Design review of the part built by this model. Coordinates are the model's own, in mm. A direction names the side the tool comes from. Coordinates: 2 decimals unless noted, no trailing zeros. Order: outer loops, then holes, each group sorted by start corner. A loop starts at its lowest first (then second) coordinate and runs counter-clockwise, first axis right, second up.
from build123d import *

# Parameters (mm, degrees)
BASE_EXTRUDE_THIN_DEPTH = 30
CHAMFER1_SIZE           = 1.4
CHAMFER1_SIZE2          = 0.808290377


with BuildPart() as part:
    # Sketch1 → Base-Extrude-Thin (new, symmetric)
    with BuildSketch(Plane.XY):
        with BuildLine():
            ThreePointArc((-0.5, 2.958039892), (0, -3), (0.5, 2.958039892))
            Line((0.5, 2.958039892), (0.3, 1.774823935))
            ThreePointArc((0.3, 1.774823935), (0, -1.8), (-0.3, 1.774823935))
            Line((-0.3, 1.774823935), (-0.5, 2.958039892))
        make_face()
    extrude(amount=BASE_EXTRUDE_THIN_DEPTH, both=True)

    # Chamfer1
    chamfer1_edges = [part.edges().sort_by_distance(p)[0] for p in [
        (0, -3, 30),
        (0, -3, -30),
    ]]
    chamfer1_side = [part.faces().sort_by_distance(p)[0] for p in [
        (0, -3, 0),
    ]]
    chamfer(chamfer1_edges, length=CHAMFER1_SIZE, length2=CHAMFER1_SIZE2, reference=chamfer1_side[0])


solid = part.part
1. Add section B-B (z = -19.5). Give the boundary of the cut face in (x, y).
2. Add section A-A (y = 0). Give the boundary of the cut face in (x, z).
3. Insertion check: pin 1 (1 mm diameter, centred on x = 1.5, z = -9.5, fed in from +Y); pin 2 (1.5 mm diameter, centred on y = -1.5, z = -14, fed in from +X). Each pin has a flat end and moves straight along its axis. Give the tip position at first contact, or say it passes through.
4. For faces 5 (the flat face through (0, -2, 30)), 6 (the flat face through (-0.4, 2.36, 0.42)), list the 3-axis set-ups (+Z, -Z, +X, -X, +Y, -Y) from which the entire face can be reached by the end or side of a thin tool; tool diameter is ignored.
5. Mouldability with a two-part tool opening along X and no side actions: class faces 1 (the cylindrical face through (0.07, -1.8, 0.42)), 2 (the flat face through (0, -2, -30)), 3 (the conical face through (-0.097, -2.319, 29.776)), 4 (the flat face through (0.4, 2.37, 0.42)) as pulls with the +X half, pulls with the -X half, needs draft (parallel to the pull), parting line crosses it, or undercut.
6. To check wall thickness, follow line 1 (X direction, y = 0, z = -5); line 2 (Y direction, x = 0, z = -5.5); line 3 (X direction, y = -0.55, z = 18). State the ranges of each line that lie inside material, in increasing order.
Solution:
1. outline: (-0.5, 2.96) arc R3 ccw (long way) to (0.5, 2.96) - (0.3, 1.77) arc R1.8 cw (long way) to (-0.3, 1.77) - close
2. outline: (-3, -28.6) - (-2.19, -30) - (-1.8, -30) - (-1.8, 30) - (-2.19, 30) - (-3, 28.6) - close; (1.8, -30) - (2.19, -30) - (3, -28.6) - (3, 28.6) - (2.19, 30) - (1.8, 30) - close
3. pin 1: stops at y = 2.83
3. pin 2: stops at x = 2.9
4. face 5: +Z, +X, -X, +Y, -Y
4. face 6: +Z, -Z, +Y
5. face 1: undercut
5. face 2: needs draft
5. face 3: parting line crosses it
5. face 4: undercut
6. line 1: x = -3 to -1.8, 1.8 to 3
6. line 2: y = -3 to -1.8
6. line 3: x = -2.95 to -1.71, 1.71 to 2.95
